from build123d import *

# Parameters (mm, degrees)
SKETCH1_W               = 82.75
SKETCH1_H               = 127
BOSS_EXTRUDE1_DEPTH     = 127
SKETCH2_R               = 6.35
CUT_EXTRUDE1_DEPTH      = 1
CUT_EXTRUDE1_DEPTH_BACK = 127
SKETCH3_W               = 28.753041512
SKETCH3_H               = 129.689601996
CUT_EXTRUDE2_DEPTH      = 127
SKETCH6_W               = 3.210142998
SKETCH6_H               = 200
CUT_EXTRUDE3_DEPTH      = 128


with BuildPart() as part:
    # Sketch1 → Boss-Extrude1 (new body)
    with BuildSketch(Plane(origin=(0, 0, 0), x_dir=(0, 0, -1), z_dir=(1, 0, 0))):
        Rectangle(SKETCH1_W, SKETCH1_H)
    extrude(amount=BOSS_EXTRUDE1_DEPTH)

    # Sketch2 → Cut-Extrude1 (cut, two sides)
    with BuildSketch(Plane(origin=(127, 0, 0), x_dir=(0, 0, -1), z_dir=(1, 0, 0))) as cut_extrude1_sk:
        with Locations((20.6875, 31.75)):
            Circle(SKETCH2_R)
        with Locations((20.6875, -31.75)):
            Circle(SKETCH2_R)
        with Locations((20.6875, 0)):
            Circle(SKETCH2_R)
    extrude(amount=CUT_EXTRUDE1_DEPTH, mode=Mode.SUBTRACT)
    extrude(cut_extrude1_sk.sketch, amount=-CUT_EXTRUDE1_DEPTH_BACK, mode=Mode.SUBTRACT)

    # Sketch3 → Cut-Extrude2 (cut)
    with BuildSketch(Plane(origin=(127, 0, 0), x_dir=(0, 0, -1), z_dir=(1, 0, 0))):
        with Locations((-53.011520756, -1.344800998)):
            Rectangle(SKETCH3_W, SKETCH3_H)
    extrude(amount=-CUT_EXTRUDE2_DEPTH, mode=Mode.SUBTRACT)

    # Sketch6 → Cut-Extrude3 (cut, through all)
    with BuildSketch(Plane(origin=(127, 0, 0), x_dir=(0, 0, -1), z_dir=(1, 0, 0))):
        with Locations((-39.450071499, -36.5)):
            Rectangle(SKETCH6_W, SKETCH6_H)
    extrude(amount=-CUT_EXTRUDE3_DEPTH, mode=Mode.SUBTRACT)


solid = part.part
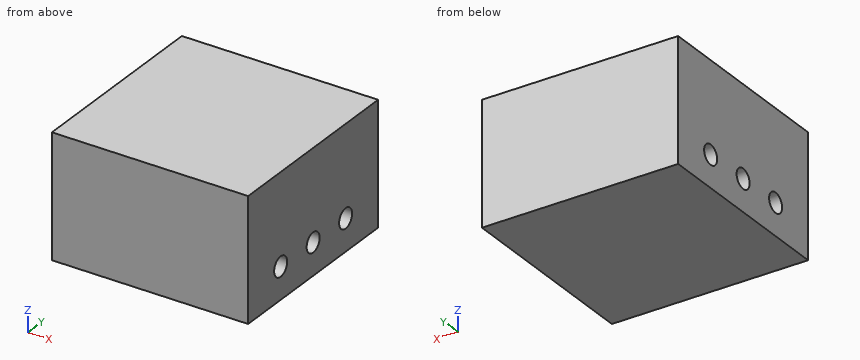
The listing builds one solid part. Answer for the finished solid, in the listing's coordinates (mm). Coordinates: 2 decimals unless noted, no trailing zeros. Write each loop counter-clockwise with the first axis right and the second up, starting at its lowest first coordinate (ties: lowest second). Pieces come first, ordered by that corner, then holes. Notation, with made-up numbers: M -10.5,30 L 39.5,30 A22 ccw 39.5,46 Z; hole C 78,23 d10. An arc over 180 degrees is marked long. Put each result on its own line as item: value. Start each with the question number.
1. A cutting plane is placed at A-A on y = 31.75. Write down the section's boundary in (x, z) (1 decimal), then the cut area to 3 significant figures.
2. A flat-ended cylindrical pin translates along its axis: P1, Ø20.5, axis at y = -31.75, z = -20.69, coming from the +X side. Find the tip coordinate at first contact, or state that the pin passes through.
3. A cutting plane is placed at B-B on x = 63. Count the separate pieces of the cut face and the enclosed holes in it, then the cut area to 3 significant figures.
4. A cutting plane is placed at C-C on z = -23.5. Write down the section's boundary in (x, y).
5. Consider line 1 (Y direction, x = 55, z = -17.5); line 2 (Z direction, x = 114.5, y = -3) (3 decimals). Determine where each line is inside the solid, lowest interval first. Write a range as from..to.
Resolved:
1. outline: M 0,-41.4 L 127,-41.4 L 127,-27 L 0,-27 Z; M 0,-14.3 L 127,-14.3 L 127,37.8 L 0,37.8 Z
1. area: 8,450 mm2
2. P1: stops at x = 127
3. separate pieces: 1
3. enclosed holes: 3
3. area: 9,680 mm2
4. outline: M 0,-63.5 L 127,-63.5 L 127,-37.44 L 0,-37.44 Z; M 0,-26.06 L 127,-26.06 L 127,-5.69 L 0,-5.69 Z; M 0,5.69 L 127,5.69 L 127,26.06 L 0,26.06 Z; M 0,37.44 L 127,37.44 L 127,63.5 L 0,63.5 Z
5. line 1: y = -63.5..-37.24, -26.26..-5.49, 5.49..26.26, 37.24..63.5
5. line 2: z = -41.375..-26.284, -15.091..37.845
